from build123d import *

# Parameters (mm, degrees)
BOSS_EXTRUDE3_DEPTH = 40
SKETCH4_R           = 11.5
SKETCH4_R_2         = 1.5
CUT_EXTRUDE1_DEPTH  = 80
SKETCH5_R           = 3.1
CUT_EXTRUDE2_DEPTH  = 40
SKETCH9_R           = 3.1
CUT_EXTRUDE3_DEPTH  = 10
SKETCH11_W          = 10
SKETCH11_H          = 80
CUT_EXTRUDE4_DEPTH  = 10


with BuildPart() as part:
    # Sketch1 → Boss-Extrude3 (new, symmetric)
    with BuildSketch(Plane.XY):
        Polygon((0, 0), (21.2, 0), (21.2, -40), (50, -40), (50, -35), (26.2, -35), (26.2, 5), (26.2, 9.75), (50, 9.5), (50, 14.5), (26.15, 14.5), (-26.15, 14.5), (-50, 14.5), (-50, 9.5), (-26.2, 9.75), (-26.2, 5), (-26.2, -35), (-50, -35), (-50, -40), (-21.2, -40), (-21.2, 0), align=None)
    extrude(amount=BOSS_EXTRUDE3_DEPTH, both=True)

    # Sketch4 → Cut-Extrude1 (cut)
    with BuildSketch(Plane(origin=(0, 14.5, 0), x_dir=(1, 0, 0), z_dir=(0, 1, 0))):
        with Locations(Location((0, 0, 0), (0, 0, 270))):
            Circle(SKETCH4_R)
        with Locations(Location((-15.5, 15.5, 0), (0, 0, 270))):
            Circle(SKETCH4_R_2)
        with Locations(Location((-15.5, -15.5, 0), (0, 0, 270))):
            Circle(SKETCH4_R_2)
        with Locations(Location((15.5, -15.5, 0), (0, 0, 270))):
            Circle(SKETCH4_R_2)
        with Locations(Location((15.5, 15.5, 0), (0, 0, 270))):
            Circle(SKETCH4_R_2)
    extrude(amount=-CUT_EXTRUDE1_DEPTH, mode=Mode.SUBTRACT)

    # Sketch5 → Cut-Extrude2 (cut)
    with BuildSketch(Plane(origin=(0, 14.5, 0), x_dir=(1, 0, 0), z_dir=(0, 1, 0))):
        with Locations(Location((33, 0, 0), (0, 0, 270))):
            Circle(SKETCH5_R)
        with Locations(Location((0, -33, 0), (0, 0, 270))):
            Circle(SKETCH5_R)
        with Locations(Location((-33, 0, 0), (0, 0, 270))):
            Circle(SKETCH5_R)
        with Locations(Location((0, 33, 0), (0, 0, 270))):
            Circle(SKETCH5_R)
    extrude(amount=-CUT_EXTRUDE2_DEPTH, mode=Mode.SUBTRACT)

    # Sketch9 → Cut-Extrude3 (cut)
    with BuildSketch(Plane.XZ.offset(40)):
        with Locations(Location((35.6, 20, 0), (0, 0, 270))):
            Circle(SKETCH9_R)
        with Locations(Location((35.6, -20, 0), (0, 0, 270))):
            Circle(SKETCH9_R)
        with Locations(Location((-35.6, -20, 0), (0, 0, 270))):
            Circle(SKETCH9_R)
        with Locations(Location((-35.6, 20, 0), (0, 0, 270))):
            Circle(SKETCH9_R)
    extrude(amount=-CUT_EXTRUDE3_DEPTH, mode=Mode.SUBTRACT)

    # Sketch11 → Cut-Extrude4 (cut)
    with BuildSketch(Plane(origin=(0, 14.5, 0), x_dir=(1, 0, 0), z_dir=(0, 1, 0))):
        with Locations((-45, 0)):
            Rectangle(SKETCH11_W, SKETCH11_H)
    extrude(amount=-CUT_EXTRUDE4_DEPTH, mode=Mode.SUBTRACT)


solid = part.part
Design review of the part built by this model. Coordinates are the model's own, in mm. A direction names the side the tool comes from. Coordinates: 2 decimals unless noted, no trailing zeros. Order: outer loops, then holes, each group sorted by start corner. A loop starts at its lowest first (then second) coordinate and runs counter-clockwise, first axis right, second up. Notation, with made-up numbers: (59, 55.5) -> (88, 55.5) arc R17 ccw to (88, 74.5) -> close; hole circle Ø3 at (35, 55). An arc over 180 degrees is marked (long way). Use one line per item in the form item = value. Start each with the question number.
(1) For probe 1 along X at (y, z) = (10.65, 0); probe 2 along X at (y, z) = (-38, 20); probe 3 along Y at (x, z) = (38, 23.5), list the stretches that pass through material, from the lowest coordinate up.
(2) Add section D-D on y = -33.5. State the section outline as (x, z) points.
(3) Add section C-C on x = 15.5. State the section outline as (y, z) points, plus the area to 3 significant figures.
(4) Add section A-A on z = -20. State the section outline as (x, y) points, plus the area to 3 significant figures.
(5) The part is to be moulded in two halves that separate along Y. For faces 4 (the flat face through (38, -35, 1)), 5 (the flat face through (-26.2, -12, 1)), 6 (the flat face through (-21.2, -20, 1)), 7 (the flat face through (-36, -40, 1)), say which applies: +Y half, -Y half, draft (parallel to the pull), parting line (faces both ways), or undercut.
(6) For faces 1 (the flat face through (-40, 12, 1)), 2 (the cylindrical face through (-15.43, 7.35, -17)), 3 (the cylindrical face through (-38.626, -37.535, -19.328)), list the 3-axis set-ups (+Z, -Z, +X, -X, +Y, -Y) from which the entire face can be reached by the end or side of a thin tool; tool diameter is ignored.
(7) Add section B-B on x = 0. State the section outline as (y, z) points, plus the area to 3 significant figures.
(8) Insertion check: pin 1 (1 mm diameter, centred on y = -26.5, z = -5.5, fed in from +X); pin 2 (8 mm diameter, centred on y = -13, z = 0, fed in from -X); pin 3 (2.5 mm diameter, centred on y = 12.5, z = 16, fed in from -X). Each pin has a flat end and moves straight along its axis. Give the tip position at first contact, or say it passes through.
Answer block:
q1.probe_1 = -40 to -36.1, -29.9 to -11.5, 11.5 to 29.9, 36.1 to 50
q1.probe_2 = -50 to -38.7, -32.5 to -21.2, 21.2 to 32.5, 38.7 to 50
q1.probe_3 = -40 to -35, 9.63 to 14.5
q2.outline = (-26.2, -40) -> (-21.2, -40) -> (-21.2, 40) -> (-26.2, 40) -> close; (21.2, -40) -> (26.2, -40) -> (26.2, 40) -> (21.2, 40) -> close
q3.outline = (0, -40) -> (14.5, -40) -> (14.5, -17) -> (0, -17) -> close; (0, -14) -> (14.5, -14) -> (14.5, 14) -> (0, 14) -> close; (0, 17) -> (14.5, 17) -> (14.5, 40) -> (0, 40) -> close
q3.area = 1,070 mm²
q4.outline = (-50, -40) -> (-38.7, -40) -> (-38.7, -35) -> (-50, -35) -> close; (-40, 9.61) -> (-26.2, 9.75) -> (-26.2, -35) -> (-32.5, -35) -> (-32.5, -40) -> (-21.2, -40) -> (-21.2, 0) -> (21.2, 0) -> (21.2, -40) -> (32.5, -40) -> (32.5, -35) -> (26.2, -35) -> (26.2, 9.75) -> (50, 9.5) -> (50, 14.5) -> (-40, 14.5) -> close; (38.7, -40) -> (50, -40) -> (50, -35) -> (38.7, -35) -> close
q4.area = 1,520 mm²
q5.face_4 = undercut
q5.face_5 = undercut
q5.face_6 = draft
q5.face_7 = -Y half
q6.face_1 = +Z, -Z, -X, +Y
q6.face_2 = +Y, -Y
q6.face_3 = -Y
q7.outline = (0, -40) -> (14.5, -40) -> (14.5, -36.1) -> (0, -36.1) -> close; (0, -29.9) -> (14.5, -29.9) -> (14.5, -11.5) -> (0, -11.5) -> close; (0, 11.5) -> (14.5, 11.5) -> (14.5, 29.9) -> (0, 29.9) -> close; (0, 36.1) -> (14.5, 36.1) -> (14.5, 40) -> (0, 40) -> close
q7.area = 647 mm²
q8.pin_1 = 26.2
q8.pin_2 = -26.2
q8.pin_3 = -40
